```python
from build123d import *

# Parameters (mm, degrees)
F0_W     = 28
F0_H     = 10
F0_W_2   = 25
F0_H_2   = 7
F1_DEPTH = 15
F2_R     = 0.75
F3_DEPTH = 10.001
F6_F1_R  = 2
F6_F2_R  = 2
F6_F3_R  = 2
F6_F4_R  = 2
F6_F5_R  = 2
F6_F6_R  = 2
F6_F7_R  = 2
F6_F8_R  = 2
F6_F9_R  = 2
F6_F10_R = 2
F6_F11_R = 2
F6_F12_R = 2


# Not quite as in the source:
# - a feature of the source that left no trace in its solid (it failed there, or was rolled back) is left out
# - a pattern or mirror of a feature is missing from the dataset's text; its kind, count and spacing are read off the source's solid


with BuildPart() as f1:
    # F0 (on Top) → F1 (new body)
    with BuildSketch(Plane.XY):
        Rectangle(F0_W, F0_H)
        Rectangle(F0_W_2, F0_H_2, mode=Mode.SUBTRACT)
    extrude(amount=F1_DEPTH)

    # F2 (on face) → F3 (cut, through all)
    with BuildSketch(Plane(origin=(0, 5, 0), x_dir=(-1, 0, 0), z_dir=(0, 1, 0))):
        with Locations((0, 7.5)):
            Circle(F2_R)
    extrude(amount=-F3_DEPTH, mode=Mode.SUBTRACT)

    # F4: sweep along a path in F4_path
    with BuildLine(Plane(origin=(14, -5, 15), x_dir=(0, -1, 0), z_dir=(0, 0, -1))) as f4_path:
        Line((0, 0), (-10, 0))
        Line((-10, 0), (-10, 28))
        Line((-10, 28), (0, 28))
        Line((0, 28), (0, 0))
    # F2 (on face) → F4 (sweep)
    with BuildSketch(Plane(origin=(0, 5, 0), x_dir=(-1, 0, 0), z_dir=(0, 1, 0))):
        Polygon((-14, 14), (-14, 15), (-15, 15), align=None)
    f4 = sweep(path=f4_path.line, transition=Transition.RIGHT)

    # F4_copies: F4 across plane
    add(f4.mirror(Plane(origin=(0, 0, 7.5), x_dir=(-1, 0, 0), z_dir=(0, 0, -1))))

    # F6: fillet of radius 2 on 12 edges, made by hand

    # F6_f1
    f6_f1_edges = [f1.edges().sort_by_distance(p)[0] for p in [
        (14, 5, 7.5),
    ]]
    fillet(f6_f1_edges, radius=F6_F1_R)

    # F6_f2
    f6_f2_edges = [f1.edges().sort_by_distance(p)[0] for p in [
        (14, -5, 7.5),
    ]]
    fillet(f6_f2_edges, radius=F6_F2_R)

    # F6_f3
    f6_f3_edges = [f1.edges().sort_by_distance(p)[0] for p in [
        (14.2071067812, -5.2071067812, 0.7928932188),
    ]]
    fillet(f6_f3_edges, radius=F6_F3_R)

    # F6_f4
    f6_f4_edges = [f1.edges().sort_by_distance(p)[0] for p in [
        (14.2071067812, 5.2071067812, 0.7928932188),
    ]]
    fillet(f6_f4_edges, radius=F6_F4_R)

    # F6_f5
    f6_f5_edges = [f1.edges().sort_by_distance(p)[0] for p in [
        (-14, 5, 7.5),
    ]]
    fillet(f6_f5_edges, radius=F6_F5_R)

    # F6_f6
    f6_f6_edges = [f1.edges().sort_by_distance(p)[0] for p in [
        (14.2071067812, -5.2071067812, 14.2071067812),
    ]]
    fillet(f6_f6_edges, radius=F6_F6_R)

    # F6_f7
    f6_f7_edges = [f1.edges().sort_by_distance(p)[0] for p in [
        (14.2071067812, 5.2071067812, 14.2071067812),
    ]]
    fillet(f6_f7_edges, radius=F6_F7_R)

    # F6_f8
    f6_f8_edges = [f1.edges().sort_by_distance(p)[0] for p in [
        (-14, -5, 7.5),
    ]]
    fillet(f6_f8_edges, radius=F6_F8_R)

    # F6_f9
    f6_f9_edges = [f1.edges().sort_by_distance(p)[0] for p in [
        (-14.2071067812, -5.2071067812, 0.7928932188),
    ]]
    fillet(f6_f9_edges, radius=F6_F9_R)

    # F6_f10
    f6_f10_edges = [f1.edges().sort_by_distance(p)[0] for p in [
        (-14.2071067812, 5.2071067812, 0.7928932188),
    ]]
    fillet(f6_f10_edges, radius=F6_F10_R)

    # F6_f11
    f6_f11_edges = [f1.edges().sort_by_distance(p)[0] for p in [
        (-14.2071067812, 5.2071067812, 14.2071067812),
    ]]
    fillet(f6_f11_edges, radius=F6_F11_R)

    # F6_f12
    f6_f12_edges = [f1.edges().sort_by_distance(p)[0] for p in [
        (-14.2071067812, -5.2071067812, 14.2071067812),
    ]]
    fillet(f6_f12_edges, radius=F6_F12_R)


solid = f1.part
```
Work out the finished part from the listing and answer in its coordinate system (mm). A direction names the side the tool comes from. Coordinates: 2 decimals unless noted, no trailing zeros. Write each loop counter-clockwise with the first axis right and the second up, starting at its lowest first coordinate (ties: lowest second). Pieces come first, ordered by that corner, then holes. Notation, with made-up numbers: (16, 1) - (58, 1) arc R6 ccw to (58, 6) - close; hole circle Ø8 at (87, 86). An arc over 180 degrees is marked (long way). Answer as a JSON object with one key per item and string values.
Q1. Given pin 1 Ø5.5 at (y, z) = (1, 8.5) entering from +X; pin 2 Ø6 at (y, z) = (-3.5, 7.5) entering from -X; pin 3 Ø4 at (x, z) = (4.5, 8.5) entering from -Y; pin 4 Ø0.9 at (x, z) = (0, 7.5) entering from -Y, each flat-ended and moving along its own axis, determine where each tip first touches the part or whether it passes through.
Results list:
{"pin 1": "stops at x = 14", "pin 2": "stops at x = -14", "pin 3": "stops at y = -5", "pin 4": "passes through"}
Q2. Find section A-A (y = -2.5). Write down the section's boundary in (x, z).
Results list:
{"outline": "(-15, 0) - (-12.5, 0) - (-12.5, 15) - (-15, 15) - (-14, 14) - (-14, 1) - close; (12.5, 0) - (15, 0) - (14, 1) - (14, 14) - (15, 15) - (12.5, 15) - close"}
Q3. Consider L1, parallel to Y at x = 11.5, z = 9.5; L2, parallel to Z at x = 0, y = 4.3; L3, parallel to X at y = 0.5, z = 1.5. Determine where each line is inside the solid, lowest interval first. Write a range as from..to.
Results list:
{"L1": "y = -5..-3.5, 3.5..5", "L2": "z = 0..6.75, 8.25..15", "L3": "x = -14..-12.5, 12.5..14"}
Q4. Which of the six approach directions +Z, -Z, +X, -X, +Y, -Y give full straight-line access (tool end or side, diameter ignored) to faces 5 (the flat face through (0, 3.5, 6)), 6 (the cylindrical face through (13.885, -4.865, 0.746)), 7 (the cylindrical face through (-13.4, -4.43, 7.59)), 8 (the cylindrical face through (13.43, 4.4, 7.59))?
Results list:
{"face 5": "+Z, -Z", "face 6": "+X, -Y", "face 7": "-X, -Y", "face 8": "+X, +Y"}
Q5. Find section B-B (x = 0). Write down the section's boundary in (y, z).
Results list:
{"outline": "(-6, 0) - (-3.5, 0) - (-3.5, 6.75) - (-5, 6.75) - (-5, 1) - close; (-6, 15) - (-5, 14) - (-5, 8.25) - (-3.5, 8.25) - (-3.5, 15) - close; (3.5, 0) - (6, 0) - (5, 1) - (5, 6.75) - (3.5, 6.75) - close; (3.5, 8.25) - (5, 8.25) - (5, 14) - (6, 15) - (3.5, 15) - close"}
Q6. For a pull along X with two mould halves and no side action, classify faces 1 (the flat face through (-12.5, 0, 7)), 2 (the cylindrical face through (-13.4, 4.43, 7.59)), 3 (the flat face through (-0.2, 5.5, 14.5)), 4 (the cylindrical face through (0.55, 4.26, 8.01)) as pulls with the +X half, pulls with the -X half, needs draft (parallel to the pull), parting line crosses it, or undercut.
Results list:
{"face 1": "undercut", "face 2": "pulls with the -X half", "face 3": "needs draft", "face 4": "undercut"}
Q7. Find section D-D (z = 7.5). Write down the section's boundary in (x, y), plus the area to 3 significant figures.
Results list:
{"outline": "(-14, -3) arc R2 ccw to (-12, -5) - (-0.75, -5) - (-0.75, -3.5) - (-12.5, -3.5) - (-12.5, 3.5) - (-0.75, 3.5) - (-0.75, 5) - (-12, 5) arc R2 ccw to (-14, 3) - close; (0.75, -5) - (12, -5) arc R2 ccw to (14, -3) - (14, 3) arc R2 ccw to (12, 5) - (0.75, 5) - (0.75, 3.5) - (12.5, 3.5) - (12.5, -3.5) - (0.75, -3.5) - close", "area": "97.1 mm^2"}
Q8. Find section C-C (z = 2.75). Write down the section's boundary in (x, y).
Results list:
{"outline": "(-14, -3) arc R2 ccw to (-12, -5) - (12, -5) arc R2 ccw to (14, -3) - (14, 3) arc R2 ccw to (12, 5) - (-12, 5) arc R2 ccw to (-14, 3) - close; hole (-12.5, -3.5) - (12.5, -3.5) - (12.5, 3.5) - (-12.5, 3.5) - close"}
